Source: CAD feature listing. Evaluate the final solid. Frame: model axes, mm. Face numbers are marked on the shaded views. A direction names the side the tool comes from. Round coordinates to 2 decimals unless told otherwise and drop trailing zeros. Order: outer loops, then holes, each group sorted by start corner. A loop starts at its lowest first (then second) coordinate and runs counter-clockwise, first axis right, second up. Notation, with made-up numbers: (-2, 27) -> (32, 27) arc R25 ccw to (32, 39) -> close; hole circle Ø3 at (15.5, 54.5). An arc over 180 degrees is marked (long way). Answer as CSV lines item,"result".
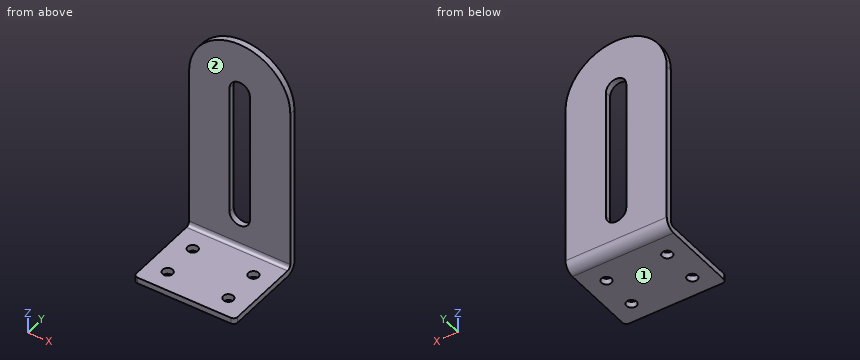
Autodesk Inventor part; units mm, degrees
ref_plane "YZ Plane" through (0, 0, 0) normal (1, 0, 0) x (0, 1, 0)
ref_plane "XZ Plane" through (0, 0, 0) normal (0, 1, 0) x (-1, 0, 0)
ref_plane "XY Plane" through (0, 0, 0) normal (0, 0, 1) x (1, 0, 0)
sketch "Boceto1" plane through (0, 0, 0) normal (0, 0, 1) x (1, 0, 0)
  line L0 (0, 0) -> (-50, 0)
  line L1 (-50, 0) -> (-50, 125)
  line L2 (0, 125) -> (0, 0)
  arc A0 (0, 125) -> (-50, 125) centre (-25, 125) ccw
  arc A1 (-20, 125) -> (-30, 125) centre (-25, 125) ccw
  line L3 (-25, 67.5) -> (-25, 60)
  arc A2 (-30, 60) -> (-20, 60) centre (-25, 60) ccw
  line L4 (-30, 60) -> (-30, 125)
  line L5 (-20, 60) -> (-20, 125)
  line L6 (0, 0) -> (-50, 0)
  line L7 (-50, 0) -> (-50, 38.1)
  line L8 (-50, 38.1) -> (0, 38.1)
  line L9 (0, 38.1) -> (0, 0)
  line L10 (-10, 28.1) -> (-40, 28.1)
  line L11 (-40, 28.1) -> (-40, 10)
  line L12 (-40, 10) -> (-10, 10)
  line L13 (-10, 10) -> (-10, 28.1)
  circle A3 centre (-40, 28.1) radius 2.5
  circle A4 centre (-10, 28.1) radius 2.5
  circle A5 centre (-40, 10) radius 2.5
  circle A6 centre (-10, 10) radius 2.5
  point P0 (-12.5, 10)
  point P1 (-10, 12.5)
  point P2 (-10, 25.6)
  point P3 (-12.5, 28.1)
  point P4 (-37.5, 28.1)
  point P5 (-40, 25.6)
  point P6 (-40, 12.5)
  point P7 (-37.5, 10)
  dimension "d2" = 10
  dimension "d3" = 65
  dimension "d4" = 10
  dimension "d5" = 38.1
  dimension "d6" = 10
  dimension "d7" = 5
  dimension "d8" = 5
  dimension "d9" = 5
  dimension "d10" = 5
extrude "Extrusión1" add sketch "Boceto1" along normal blind 3 contours L0 L1 L8 L2 | L8 L1 A0 L2 | L5 A2 L4 A1 | A3 L11 L10 | L10 L11 A3 | L10 A4 L13 A6 L12 A5 L11 A3 | A4 L13 L10 | L10 L13 A4 | A5 L12 L11 | L11 L12 A5 | A6 L12 L13 | L13 L12 A6
fillet "Empalme1" radius 2 2 edges at (0, 0, 1.5) (-50, 0, 1.5)
extrude "Extrusión2" cut sketch "Boceto1" along normal blind 3 contours L5 A2 L4 A1 | A3 L11 L10 | L10 L11 A3 | A4 L13 L10 | L10 L13 A4 | A5 L12 L11 | L11 L12 A5 | A6 L12 L13 | L13 L12 A6
bend part "Pieza de plegado1" radius 5 angle 90 line through (-50, 38.1, 0) along (1, 0, 0) centre toward (0, 0, 1) moving side (0, 1, 0) both sides no
1. Line query: L1, parallel to X at y = 28, z = 1; L2, parallel to Y at x = -40, z = 2.45; L3, parallel to Y at x = -10, z = 2. Output: solid intervals per line, ascending. Write a range as [from, to].
Results below:
L1,"[-50, -42.5], [-37.5, -12.5], [-7.5, 0]"
L2,"[0, 7.5], [12.5, 25.6], [30.6, 42.4]"
L3,"[0, 7.5], [12.5, 25.6], [30.6, 42.1]"
2. Section query B-B on z = 46. Return loops of the section in (x, y), and give its area (3 significant figures).
Results below:
outline,"(-50, 40.1) -> (-30, 40.1) -> (-30, 43.1) -> (-50, 43.1) -> close; (-20, 40.1) -> (0, 40.1) -> (0, 43.1) -> (-20, 43.1) -> close"
area,"120 mm2"
3. Section query C-C on x = -25. Return loops of the section in (y, z), and give its area (3 significant figures).
Results below:
outline,"(0, 0) -> (38.1, 0) arc R5 ccw to (43.1, 5) -> (43.1, 14.05) -> (40.1, 14.05) -> (40.1, 5) arc R2 cw to (38.1, 3) -> (0, 3) -> close; (40.1, 89.05) -> (43.1, 89.05) -> (43.1, 109.05) -> (40.1, 109.05) -> close"
area,"218 mm2"
4. Pin query (flat end, axial travel): pin 1 (6.5 mm diameter, centred on x = -10, y = 28.1, fed in from +Z); pin 2 (5 mm diameter, centred on x = -42, z = 95, fed in from -Y). Return the tip coordinate at first contact, or that it passes through.
Results below:
pin 1,"z = 3"
pin 2,"y = 40.1"
5. Section query A-A on y = 10. Return loops of the section in (x, z).
Results below:
outline,"(-50, 0) -> (-42.5, 0) -> (-42.5, 3) -> (-50, 3) -> close; (-37.5, 0) -> (-12.5, 0) -> (-12.5, 3) -> (-37.5, 3) -> close; (-7.5, 0) -> (0, 0) -> (0, 3) -> (-7.5, 3) -> close"
6. Section query D-D on x = -10. Return loops of the section in (y, z).
Results below:
outline,"(0, 0) -> (7.5, 0) -> (7.5, 3) -> (0, 3) -> close; (12.5, 0) -> (25.6, 0) -> (25.6, 3) -> (12.5, 3) -> close; (30.6, 0) -> (38.1, 0) arc R5 ccw to (43.1, 5) -> (43.1, 104.05) -> (40.1, 104.05) -> (40.1, 5) arc R2 cw to (38.1, 3) -> (30.6, 3) -> close"
7. Reachability of the marked faces 1 and 2 from +Z, -Z, +X, -X, +Y, -Y: full face, straight path, thin tool, end or side. Return the list, or none.
Results below:
face 1,"-Z, +X, -X, +Y, -Y"
face 2,"+Z, +X, -X, -Y"
